Can you work these out from the model? Positions are in its coordinate system, mm. A direction names the side the tool comes from. Give positions to 0.01 mm unless a question says otherwise; leave off trailing zeros. Loops run counter-clockwise (first coordinate to the right, second up) from the corner with the lowest first, then second, coordinate; pieces in that order, holes last. Notation, with made-up numbers: (62.5, 18.25) - (114.5, 18.25) arc R4 cw to (114.5, 25.25) - close; hole circle Ø10 at (9, 22.5). An arc over 180 degrees is marked (long way). Write item = value, one per line.
from build123d import *

# Parameters (mm, degrees)
SKETCH1_R                   = 6.35
BOSS_EXTRUDE1_DEPTH         = 3.175
F_4_CLEARANCE_HOLE1_D       = 2.9464
CUT_EXTRUDE1_REACH          = 33.591
SKETCH11_W                  = 3.175
SKETCH11_H                  = 6.918259867
CIRPATTERN2_COUNT           = 4
CIRPATTERN2_COPY_1_REACH    = 33.591
CIRPATTERN2_COPY_1_SKETCH_W = 3.175
CIRPATTERN2_COPY_1_SKETCH_H = 6.918259867
CIRPATTERN2_COPY_2_REACH    = 33.591
CIRPATTERN2_COPY_2_SKETCH_W = 3.175
CIRPATTERN2_COPY_2_SKETCH_H = 6.918259867
CIRPATTERN2_COPY_3_REACH    = 33.591
CIRPATTERN2_COPY_3_SKETCH_W = 3.175
CIRPATTERN2_COPY_3_SKETCH_H = 6.918259867
CIRPATTERN2_COPY_4_REACH    = 33.591
CIRPATTERN2_COPY_4_SKETCH_W = 3.175
CIRPATTERN2_COPY_4_SKETCH_H = 6.918259867
CIRPATTERN2_COPY_5_REACH    = 33.591
CIRPATTERN2_COPY_5_SKETCH_W = 3.175
CIRPATTERN2_COPY_5_SKETCH_H = 6.918259867
CIRPATTERN2_COPY_6_REACH    = 33.591
CIRPATTERN2_COPY_6_SKETCH_W = 3.175
CIRPATTERN2_COPY_6_SKETCH_H = 6.918259867


with BuildPart() as part:
    # Sketch1 → Boss-Extrude1 (new body)
    with BuildSketch(Plane(origin=(0, 0, 0), x_dir=(1, 0, 0), z_dir=(0, 1, 0))):
        with BuildLine():
            Line((-3.175, 21.997045256), (-3.175, 15.554259867))
            ThreePointArc((-3.175, 15.554259867), (-11.225320151, 11.225320151), (-15.554259867, 3.175))
            Line((-15.554259867, 3.175), (-21.997045256, 3.175))
            ThreePointArc((-21.997045256, 3.175), (-22.225, 0), (-21.997045256, -3.175))
            Line((-21.997045256, -3.175), (-15.554259867, -3.175))
            ThreePointArc((-15.554259867, -3.175), (-11.225320151, -11.225320151), (-3.175, -15.554259867))
            Line((-3.175, -15.554259867), (-3.175, -21.997045256))
            ThreePointArc((-3.175, -21.997045256), (0, -22.225), (3.175, -21.997045256))
            Line((3.175, -21.997045256), (3.175, -15.554259867))
            ThreePointArc((3.175, -15.554259867), (11.225320151, -11.225320151), (15.554259867, -3.175))
            Line((15.554259867, -3.175), (21.997045256, -3.175))
            ThreePointArc((21.997045256, -3.175), (22.225, 0), (21.997045256, 3.175))
            Line((21.997045256, 3.175), (15.554259867, 3.175))
            ThreePointArc((15.554259867, 3.175), (11.225320151, 11.225320151), (3.175, 15.554259867))
            Line((3.175, 15.554259867), (3.175, 21.997045256))
            ThreePointArc((3.175, 21.997045256), (0, 22.225), (-3.175, 21.997045256))
        make_face()
        with Locations(Location((0, 0, 0), (0, 0, 270))):
            Circle(SKETCH1_R, mode=Mode.SUBTRACT)
    extrude(amount=BOSS_EXTRUDE1_DEPTH)

    # #4 Clearance Hole1 (through all)
    with Locations(Plane(origin=(-5.152902703, 3.175, -13.741681739), x_dir=(1, 0, 0), z_dir=(0, 1, 0))):
        with Locations((5.152902703, -1.041681739)):
            f_4_clearance_hole1 = Hole(F_4_CLEARANCE_HOLE1_D / 2)

    # Sketch11 → Cut-Extrude1 (cut, up to next)
    with BuildSketch(Plane(origin=(0, 3.175, 0), x_dir=(1, 0, 0), z_dir=(0, 1, 0)), mode=Mode.PRIVATE) as cut_extrude1_sk1:
        with Locations((-4.7625, 12.095129934)):
            Rectangle(SKETCH11_W, SKETCH11_H)
    cut_extrude1_tool1 = extrude(cut_extrude1_sk1.sketch, amount=-CUT_EXTRUDE1_REACH, mode=Mode.PRIVATE) & part.part
    cut_extrude1 = cut_extrude1_tool1.solids().sort_by_distance((-4.7625, 3.175, -12.09513))[0]
    add(cut_extrude1, mode=Mode.SUBTRACT)

    # Mirror1: Cut-Extrude1 across plane
    add(cut_extrude1.mirror(Plane(origin=(0, 0, 0), x_dir=(0, 0, 1), z_dir=(1, 0, 0))), mode=Mode.SUBTRACT)

    # CirPattern2: #4 Clearance Hole1 ×4 about axis
    cirpattern2_axis = Axis((0, 0, 0), (0, 1, 0))
    for i in range(1, CIRPATTERN2_COUNT):
        add(f_4_clearance_hole1.rotate(cirpattern2_axis, i * 360 / CIRPATTERN2_COUNT), mode=Mode.SUBTRACT)

    # CirPattern2 copy 1 sketch → CirPattern2 copy 1 (cut, up to next)
    with BuildSketch(Plane.ZX.offset(3.175), mode=Mode.PRIVATE) as cirpattern2_copy_1_sk1:
        with Locations((-4.7625, -12.095129934)):
            Rectangle(CIRPATTERN2_COPY_1_SKETCH_W, CIRPATTERN2_COPY_1_SKETCH_H)
    cirpattern2_copy_1_tool1 = extrude(cirpattern2_copy_1_sk1.sketch, amount=-CIRPATTERN2_COPY_1_REACH, mode=Mode.PRIVATE) & part.part
    add(cirpattern2_copy_1_tool1.solids().sort_by_distance((-12.09513, 3.175, -4.7625))[0], mode=Mode.SUBTRACT)

    # CirPattern2 copy 2 sketch → CirPattern2 copy 2 (cut, up to next)
    with BuildSketch(Plane(origin=(0, 3.175, 0), x_dir=(1, 0, 0), z_dir=(0, 1, 0)), mode=Mode.PRIVATE) as cirpattern2_copy_2_sk1:
        with Locations((-4.7625, -12.095129934)):
            Rectangle(CIRPATTERN2_COPY_2_SKETCH_W, CIRPATTERN2_COPY_2_SKETCH_H)
    cirpattern2_copy_2_tool1 = extrude(cirpattern2_copy_2_sk1.sketch, amount=-CIRPATTERN2_COPY_2_REACH, mode=Mode.PRIVATE) & part.part
    add(cirpattern2_copy_2_tool1.solids().sort_by_distance((-4.7625, 3.175, 12.09513))[0], mode=Mode.SUBTRACT)

    # CirPattern2 copy 3 sketch → CirPattern2 copy 3 (cut, up to next)
    with BuildSketch(Plane(origin=(0, 3.175, 0), x_dir=(0, 0, -1), z_dir=(0, 1, 0)), mode=Mode.PRIVATE) as cirpattern2_copy_3_sk1:
        with Locations((-4.7625, -12.095129934)):
            Rectangle(CIRPATTERN2_COPY_3_SKETCH_W, CIRPATTERN2_COPY_3_SKETCH_H)
    cirpattern2_copy_3_tool1 = extrude(cirpattern2_copy_3_sk1.sketch, amount=-CIRPATTERN2_COPY_3_REACH, mode=Mode.PRIVATE) & part.part
    add(cirpattern2_copy_3_tool1.solids().sort_by_distance((12.09513, 3.175, 4.7625))[0], mode=Mode.SUBTRACT)

    # CirPattern2 copy 4 sketch → CirPattern2 copy 4 (cut, up to next)
    with BuildSketch(Plane(origin=(0, 3.175, 0), x_dir=(0, 0, -1), z_dir=(0, 1, 0)), mode=Mode.PRIVATE) as cirpattern2_copy_4_sk1:
        with Locations((-4.7625, 12.095129934)):
            Rectangle(CIRPATTERN2_COPY_4_SKETCH_W, CIRPATTERN2_COPY_4_SKETCH_H)
    cirpattern2_copy_4_tool1 = extrude(cirpattern2_copy_4_sk1.sketch, amount=-CIRPATTERN2_COPY_4_REACH, mode=Mode.PRIVATE) & part.part
    add(cirpattern2_copy_4_tool1.solids().sort_by_distance((-12.09513, 3.175, 4.7625))[0], mode=Mode.SUBTRACT)

    # CirPattern2 copy 5 sketch → CirPattern2 copy 5 (cut, up to next)
    with BuildSketch(Plane(origin=(0, 3.175, 0), x_dir=(-1, 0, 0), z_dir=(0, 1, 0)), mode=Mode.PRIVATE) as cirpattern2_copy_5_sk1:
        with Locations((-4.7625, 12.095129934)):
            Rectangle(CIRPATTERN2_COPY_5_SKETCH_W, CIRPATTERN2_COPY_5_SKETCH_H)
    cirpattern2_copy_5_tool1 = extrude(cirpattern2_copy_5_sk1.sketch, amount=-CIRPATTERN2_COPY_5_REACH, mode=Mode.PRIVATE) & part.part
    add(cirpattern2_copy_5_tool1.solids().sort_by_distance((4.7625, 3.175, 12.09513))[0], mode=Mode.SUBTRACT)

    # CirPattern2 copy 6 sketch → CirPattern2 copy 6 (cut, up to next)
    with BuildSketch(Plane.ZX.offset(3.175), mode=Mode.PRIVATE) as cirpattern2_copy_6_sk1:
        with Locations((-4.7625, 12.095129934)):
            Rectangle(CIRPATTERN2_COPY_6_SKETCH_W, CIRPATTERN2_COPY_6_SKETCH_H)
    cirpattern2_copy_6_tool1 = extrude(cirpattern2_copy_6_sk1.sketch, amount=-CIRPATTERN2_COPY_6_REACH, mode=Mode.PRIVATE) & part.part
    add(cirpattern2_copy_6_tool1.solids().sort_by_distance((12.09513, 3.175, -4.7625))[0], mode=Mode.SUBTRACT)


solid = part.part
Q1. For pin 1 (1 mm diameter, centred on x = -12.5, y = 2, fed in from -Z); pin 2 (1.6 mm diameter, centred on x = 5.5, y = 2, fed in from +Z); pin 3 (1.6 mm diameter, centred on x = 12.5, y = 2, fed in from +Z); pin 4 (1.8 mm diameter, centred on x = -12.7, z = 0, fed in from +Y), each with a flat end and sliding along its axis, tell me the tip position at first contact or that it passes through.
Output:
pin_1 = -10.39
pin_2 = 8.64
pin_3 = 10.73
pin_4 = through
Q2. Imagine slicing it at A-A, the plane x = 0. Write out the boundary of the cut face in (y, z) (3 decimals), then the cut area to 3 significant figures.
Output:
outline = (0, -22.225) - (3.175, -22.225) - (3.175, -14.173) - (0, -14.173) - close; (0, -11.227) - (3.175, -11.227) - (3.175, -6.35) - (0, -6.35) - close; (0, 6.35) - (3.175, 6.35) - (3.175, 11.227) - (0, 11.227) - close; (0, 14.173) - (3.175, 14.173) - (3.175, 22.225) - (0, 22.225) - close
area = 82.1 mm2
Q3. Which directions (+Z, -Z, +X, -X, +Y, -Y) give clear straight access to the entire face, cutting with the end or side of a thin tool? Please do faces 5 (the flat face through (5, 2, -8.636)), 6 (the flat face through (12, 2, 6.35)), 7 (the flat face through (-7, 0, 0)), 8 (the flat face through (5, 2, 8.636)), 9 (the flat face through (-15, 2, -3.175)).
Output:
face_5 = -Z, +Y, -Y
face_6 = +X, +Y, -Y
face_7 = +Z, -Z, +X, -X, -Y
face_8 = +Z, +Y, -Y
face_9 = -X, +Y, -Y
Q4. I need wall thicknesses on L1, parallel to X at y = 1.7, z = -13.5 (3 decimals); L2, parallel to X at y = 0.8, z = -11.5 (3 decimals). Which ranges of each line are inside material? Lowest first, please.
Output:
L1 = -8.353 to -6.35, -3.175 to -1.237, 1.237 to 3.175, 6.35 to 8.353
L2 = -10.944 to -6.35, -3.175 to -0.855, 0.855 to 3.175, 6.35 to 10.944
Q5. We'd pull the mould along Z, two halves only. Please class faces 1 (the cylindrical face through (-11.28, 1.57, 11.17)), 2 (the flat face through (-5, 2, -8.636)), 3 (the flat face through (8.636, 2, -5)), 4 (the flat face through (12, 2, -6.35)): released by +Z, released by -Z, zero draft, split by the parting line, or undercut.
Output:
face_1 = released by +Z
face_2 = released by -Z
face_3 = undercut
face_4 = undercut
Q6. Imagine slicing it at B-B, the plane z = 0. Write out the boundary of the cut face in (x, y) (3 decimals).
Output:
outline = (-22.225, 0) - (-14.173, 0) - (-14.173, 3.175) - (-22.225, 3.175) - close; (-11.227, 0) - (-6.35, 0) - (-6.35, 3.175) - (-11.227, 3.175) - close; (6.35, 0) - (11.227, 0) - (11.227, 3.175) - (6.35, 3.175) - close; (14.173, 0) - (22.225, 0) - (22.225, 3.175) - (14.173, 3.175) - close
Q7. Imagine slicing it at D-D, the plane x = -4.5. Write out the boundary of the cut face in (y, z) (3 decimals).
Output:
outline = (0, -8.636) - (3.175, -8.636) - (3.175, -4.48) - (0, -4.48) - close; (0, 4.48) - (3.175, 4.48) - (3.175, 8.636) - (0, 8.636) - close
Q8. Imagine slicing it at C-C, the plane z = 5.5. Write out the boundary of the cut face in (x, y) (3 decimals), then the cut area to 3 significant figures.
Output:
outline = (-8.636, 0) - (-3.174, 0) - (-3.174, 3.175) - (-8.636, 3.175) - close; (3.174, 0) - (8.636, 0) - (8.636, 3.175) - (3.174, 3.175) - close
area = 34.7 mm2
